```python
from build123d import *

# Parameters (mm, degrees)
SKETCH_2_W          = 6.5
SKETCH_2_H          = 6.4
EXTRUDE_1_DEPTH     = 6.4
SKETCH_5_R          = 2.7
CUT_EXTRUDE_1_DEPTH = 5


with BuildPart() as part:
    # 草图1 → 旋转1 (revolve)
    with BuildSketch(Plane.XY, mode=Mode.PRIVATE) as revolve_1_sk:
        with BuildLine():
            Line((0, 0), (-3.036670619, 0))
            Line((-3.036670619, 0), (-3.036670619, 1.125720416))
            Line((-3.036670619, 1.125720416), (-4, 1.125720416))
            Line((-4, 1.125720416), (-4, 2))
            Line((-4, 2), (-3.6, 2))
            Line((-3.6, 2), (-3.6, 4.5))
            Line((-3.6, 4.5), (-4, 4.5))
            Line((-4, 4.5), (-4, 8))
            Line((-4, 8), (-5, 8))
            Line((-5, 8), (-5, 25))
            add(Edge.make_bspline(
                [(-5, 25), (-4.722166372, 30.033496439), (-3.774780509, 37.406959566), (-3.370776113, 40.075486719), (-1.977019792, 43.14029628), (-1.896061892, 44.030808648), (0, 44.5)],
                knots=[0, 0, 0, 0, 0.132032401, 0.478362498, 0.569488384, 1, 1, 1, 1], degree=3))
            Line((0, 44.5), (0, 0))
        make_face()
    revolve(revolve_1_sk.sketch.rotate(Axis((0, -22.695068061, 0), (0, 1, 0)), 270), axis=Axis((0, -22.695068061, 0), (0, 1, 0)))

    # 草图2 → 凸台-拉伸1 (add)
    with BuildSketch(Plane.XZ):
        Rectangle(SKETCH_2_W, SKETCH_2_H)
    extrude(amount=EXTRUDE_1_DEPTH)

    # 草图4 → 旋转4 (revolve)
    with BuildSketch(Plane.XY):
        Polygon((-3.25, -0.1), (-4.75, -0.1), (-4.75, 1.05), (-10.75, 1.05), (-10.75, 0.7), (-13.25, 0.7), (-13.25, -3.2), (-3.25, -3.2), align=None)
    revolve(axis=Axis((-3.25, -3.2, 0), (-1, 0, 0)))

    # 草图5 → 切除-拉伸1 (cut)
    with BuildSketch(Plane.ZY.offset(13.25)):
        with Locations(Location((0, -3.2, 0), (0, 0, 270))):
            Circle(SKETCH_5_R)
    extrude(amount=-CUT_EXTRUDE_1_DEPTH, mode=Mode.SUBTRACT)


solid = part.part
```
The model under review builds one solid part; all positions refer to its coordinate system, in mm. A direction names the side the tool comes from. Coordinates: 2 decimals unless noted, no trailing zeros. Write each loop counter-clockwise with the first axis right and the second up, starting at its lowest first coordinate (ties: lowest second). Pieces come first, ordered by that corner, then holes. Notation, with made-up numbers: (83.5, -2) -> (111.5, -2) arc R20 cw to (111.5, 9) -> close; hole circle Ø9 at (-25, 70.25). An arc over 180 degrees is marked (long way). One line per item, written item: value. Start each with the question number.
Q1. Add section B-B, the plane y = 22. Give the boundary of the cut face in (x, z).
Q2. The part is to be moulded in two halves that separate along Y. For faces 4 (the face through (-4.75, 0, 1)), 5 (the face through (-12.02, 0.52, -1.17)), 6 (the face through (0, -3, 3.2)), say which applies: +Y half, -Y half, draft (parallel to the pull), parting line (faces both ways), or undercut.
Q3. Clearance check with flat-ended pins moving along their axes: P1, Ø1.5, axis at y = 30.5, z = -2.5, coming from the +X side; P2, Ø3, axis at x = -8.5, z = 3, coming from the +Y side; P3, Ø4, axis at y = -3, z = 0.5, coming from the -X side. State where each tip first meets the part, or that it passes through.
Q4. To check wall thickness, follow probe 1 along Z at (x, y) = (-11.3, -3.2); probe 2 along X at (y, z) = (31.5, -2.25); probe 3 along X at (y, z) = (33.5, -1.5). State the ranges of each line that lie inside material, in increasing order.
Q5. For faces 1 (the face through (4.88, 16.62, 1.08)), 2 (the face through (-8.25, -3, 0)), 3 (the face through (3.905, 6.274, 0.867)), list the 3-axis set-ups (+Z, -Z, +X, -X, +Y, -Y) from which the entire face can be reached by the end or side of a thin tool; tool diameter is ignored.
Q6. Add section A-A, the plane y = -3.2. Give the boundary of the cut face in (x, z).
Response:
1. outline: circle Ø10 at (0, 0)
2. face 4: undercut
2. face 5: parting line
2. face 6: draft
3. P1: x = 4.28
3. P2: y = 0.78
3. P3: x = -8.25
4. probe 1: -3.9 to -2.7, 2.7 to 3.9
4. probe 2: -3.91 to 3.91
4. probe 3: -4 to 4
5. face 1: +Y
5. face 2: -X
5. face 3: none
6. outline: (-13.25, -3.9) -> (-10.75, -3.9) -> (-10.75, -4.25) -> (-4.75, -4.25) -> (-4.75, -3.1) -> (-3.25, -3.1) -> (-3.25, -3.2) -> (3.25, -3.2) -> (3.25, 3.2) -> (-3.25, 3.2) -> (-3.25, 3.1) -> (-4.75, 3.1) -> (-4.75, 4.25) -> (-10.75, 4.25) -> (-10.75, 3.9) -> (-13.25, 3.9) -> (-13.25, 2.7) -> (-8.25, 2.7) -> (-8.25, -2.7) -> (-13.25, -2.7) -> close
